For this review, take the finished solid that the model builds, in its own axes (mm). A direction names the side the tool comes from. Coordinates: 2 decimals unless noted, no trailing zeros. Loops run counter-clockwise (first coordinate to the right, second up) from the corner with the lowest first, then second, coordinate; pieces in that order, holes last. Notation, with made-up numbers: (59, -27.5) - (81, -27.5) arc R32 cw to (81, 1.5) - close; hole circle Ø10 at (30, 6.25). An arc over 180 degrees is marked (long way). One line per item, written item: value. Start each with the question number.
1. For faces 4 (the face through (-84.74, 46.29, 0.99)), 5 (the face through (-75.315, 91, 1)), 6 (the face through (-5.815, 91, 1)), 7 (the face through (-75.315, -1, 1)), 8 (the face through (-5.815, -1, 1)), list the 3-axis set-ups (+Z, -Z, +X, -X, +Y, -Y) from which the entire face can be reached by the end or side of a thin tool; tool diameter is ignored.
2. The part is to be moulded in two halves that separate along Y. For faces 1 (the face through (-39.28, 1.36, 0.99)), 2 (the face through (-81.21, 4.354, 0.986)), 3 (the face through (-41, 46, 2)), say which applies: released by +Y, released by -Y, zero draft, split by the parting line, or undercut.
3. Take a section at A-A, the plane x = -81. State the section outline as (y, z) points, and give its area (3 significant figures).
4. Take a section at B-B, the plane z = 1.35. Count the separate pieces of the cut face and the enclosed holes in it, and give its area (3 significant figures).
5. Insertion check: pin 1 (0.6 mm diameter, centred on y = 90.5, z = 1, fed in from -X); pin 2 (1 mm diameter, centred on x = 5.5, z = 1, fed in from -Y); pin 3 (0.8 mm diameter, centred on x = -78.5, z = 1, fed in from +Y). Each pin has a flat end and moves straight along its axis. Give the tip position at first contact, or say it passes through.
6. To check wall thickness, follow line 1 (X direction, y = 45, z = 0.35); line 2 (Y direction, x = -41.5, z = 1.7); line 3 (Y direction, x = -78.5, z = 1.1). State the ranges of each line that lie inside material, in increasing order. Write a range as from..to.
```python
from build123d import *

# Parameters (mm, degrees)
SKETCH2_R           = 1.35
BOSS_EXTRUDE1_DEPTH = 2


with BuildPart() as part:
    # Sketch2 → Boss-Extrude1 (new body)
    with BuildSketch(Plane.XY):
        with BuildLine():
            Line((-5.815342674, -2.04814307), (-5.815342674, 0.45185693))
            ThreePointArc((-5.815342674, 0.45185693), (-4.936663017, 2.573177274), (-2.815342674, 3.45185693))
            Line((-2.815342674, 3.45185693), (-2.065342674, 3.45185693))
            ThreePointArc((-2.065342674, 3.45185693), (0.05597767, 4.330536587), (0.934657326, 6.45185693))
            Line((0.934657326, 6.45185693), (0.934657326, 7.20185693))
            ThreePointArc((0.934657326, 7.20185693), (1.813336983, 9.323177274), (3.934657326, 10.20185693))
            Line((3.934657326, 10.20185693), (6.434657326, 10.20185693))
            Line((6.434657326, 10.20185693), (6.43465612, 79.70185693))
            Line((6.43465612, 79.70185693), (3.93465612, 79.70185693))
            ThreePointArc((3.93465612, 79.70185693), (1.813335776, 80.580536587), (0.93465612, 82.70185693))
            Line((0.93465612, 82.70185693), (0.93465612, 83.45185693))
            ThreePointArc((0.93465612, 83.45185693), (0.055976464, 85.573177274), (-2.06534388, 86.45185693))
            Line((-2.06534388, 86.45185693), (-2.81534388, 86.45185693))
            ThreePointArc((-2.81534388, 86.45185693), (-4.936664224, 87.330536587), (-5.81534388, 89.45185693))
            Line((-5.81534388, 89.45185693), (-5.81534388, 91.95185693))
            Line((-5.81534388, 91.95185693), (-75.31534388, 91.95185693))
            Line((-75.31534388, 91.95185693), (-75.31534388, 89.45185693))
            ThreePointArc((-75.31534388, 89.45185693), (-76.194023536, 87.330536587), (-78.31534388, 86.45185693))
            Line((-78.31534388, 86.45185693), (-79.06534388, 86.45185693))
            ThreePointArc((-79.06534388, 86.45185693), (-81.186664224, 85.573177274), (-82.06534388, 83.45185693))
            Line((-82.06534388, 83.45185693), (-82.06534388, 82.70185693))
            ThreePointArc((-82.06534388, 82.70185693), (-82.944023536, 80.580536587), (-85.06534388, 79.70185693))
            Line((-85.06534388, 79.70185693), (-87.56534388, 79.70185693))
            Line((-87.56534388, 79.70185693), (-87.565342674, 10.20185693))
            Line((-87.565342674, 10.20185693), (-85.065342674, 10.20185693))
            ThreePointArc((-85.065342674, 10.20185693), (-82.94402233, 9.323177274), (-82.065342674, 7.20185693))
            Line((-82.065342674, 7.20185693), (-82.065342674, 6.45185693))
            ThreePointArc((-82.065342674, 6.45185693), (-81.186663017, 4.330536587), (-79.065342674, 3.45185693))
            Line((-79.065342674, 3.45185693), (-78.315342674, 3.45185693))
            ThreePointArc((-78.315342674, 3.45185693), (-76.19402233, 2.573177274), (-75.315342674, 0.45185693))
            Line((-75.315342674, 0.45185693), (-75.315342674, -2.04814307))
            Line((-75.315342674, -2.04814307), (-5.815342674, -2.04814307))
        make_face()
        with Locations((-40.56534404, 88.95185693)):
            Circle(SKETCH2_R, mode=Mode.SUBTRACT)
        with Locations((-84.565343277, 44.95185693)):
            Circle(SKETCH2_R, mode=Mode.SUBTRACT)
        with Locations((3.434656723, 44.95185693)):
            Circle(SKETCH2_R, mode=Mode.SUBTRACT)
        with Locations((-40.565342513, 0.95185693)):
            Circle(SKETCH2_R, mode=Mode.SUBTRACT)
    extrude(amount=BOSS_EXTRUDE1_DEPTH)


solid = part.part
```
Solutions:
1. face 4: +Z, -Z
1. face 5: +Z, -Z, -X, +Y
1. face 6: +Z, -Z, +X, +Y
1. face 7: +Z, -Z, -X, -Y
1. face 8: +Z, -Z, +X, -Y
2. face 1: undercut
2. face 2: released by -Y
2. face 3: zero draft
3. outline: (4.16, 0) - (85.74, 0) - (85.74, 2) - (4.16, 2) - close
3. area: 163 mm2
4. separate pieces: 1
4. enclosed holes: 4
4. area: 8,400 mm2
5. pin 1: x = -75.32
5. pin 2: y = 10.2
5. pin 3: y = 86.46
6. line 1: -87.57..-85.91, -83.22..2.09, 4.78..6.43
6. line 2: -2.05..-0.02, 1.93..87.98, 89.93..91.95
6. line 3: 3.45..86.45
